Source: CAD feature listing. Evaluate the final solid. Frame: model axes, mm. A direction names the side the tool comes from. Give positions to 0.01 mm unless a question says otherwise; leave off trailing zeros. Write each loop counter-clockwise with the first axis right and the second up, starting at its lowest first coordinate (ties: lowest second). Pieces come first, ordered by that corner, then holes. Notation, with made-up numbers: (75, 66) -> (120, 66) arc R25 ccw to (120, 99) -> close; hole circle Ø4 at (-23.75, 65). An arc over 180 degrees is marked (long way). Write item = value, one per line.
from build123d import *

# Parameters (mm, degrees)
SKETCH006_W     = 44
SKETCH006_H     = 43
SKETCH006_W_2   = 24
SKETCH006_H_2   = 23
PAD007_DEPTH    = 3
SKETCH007_W     = 44
SKETCH007_H     = 43
SKETCH007_W_2   = 38
SKETCH007_H_2   = 37
PAD008_DEPTH    = 40
CHAMFER007_SIZE = 1.9
CHAMFER008_SIZE = 0.4


with BuildPart() as part:
    # Sketch006 → Pad007 (new body)
    with BuildSketch(Plane.XY):
        Rectangle(SKETCH006_W, SKETCH006_H)
        Rectangle(SKETCH006_W_2, SKETCH006_H_2, mode=Mode.SUBTRACT)
    extrude(amount=PAD007_DEPTH)

    # Sketch007 (on Face9 of Pad007) → Pad008 (join)
    with BuildSketch(Plane(origin=(0, 0, 0), x_dir=(1, 0, 0), z_dir=(0, 0, -1))):
        Rectangle(SKETCH007_W, SKETCH007_H)
        Rectangle(SKETCH007_W_2, SKETCH007_H_2, mode=Mode.SUBTRACT)
    extrude(amount=PAD008_DEPTH)

    # Chamfer007
    chamfer007_edges = [part.edges().sort_by_distance(p)[0] for p in [
        (0, -11.5, 0),
        (12, 0, 0),
        (0, 11.5, 0),
        (-12, 0, 0),
    ]]
    chamfer(chamfer007_edges, length=CHAMFER007_SIZE)

    # Chamfer008
    chamfer008_edges = [part.edges().sort_by_distance(p)[0] for p in [
        (-22, 0, -40),
        (0, 21.5, -40),
        (22, 0, -40),
        (0, -21.5, -40),
        (-19, 0, -40),
        (0, 18.5, -40),
        (19, 0, -40),
        (0, -18.5, -40),
        (22, 21.5, -18.5),
        (-22, 21.5, -18.5),
        (0, 21.5, 3),
        (-22, 0, 3),
        (0, -21.5, 3),
        (22, 0, 3),
        (-12, 0, 3),
        (0, -11.5, 3),
        (12, 0, 3),
        (0, 11.5, 3),
        (-22, -21.5, -18.5),
        (22, -21.5, -18.5),
    ]]
    chamfer(chamfer008_edges, length=CHAMFER008_SIZE)


solid = part.part
1) Cut plane A-A (y = 4.5). Return the cut outline in (x, z).
Computed:
outline = (-22, -39.6) -> (-21.6, -40) -> (-19.4, -40) -> (-19, -39.6) -> (-19, 0) -> (-13.9, 0) -> (-12, 1.9) -> (-12, 2.6) -> (-12.4, 3) -> (-21.6, 3) -> (-22, 2.6) -> close; (12, 1.9) -> (13.9, 0) -> (19, 0) -> (19, -39.6) -> (19.4, -40) -> (21.6, -40) -> (22, -39.6) -> (22, 2.6) -> (21.6, 3) -> (12.4, 3) -> (12, 2.6) -> close
2) Cut plane C-C (z = -2). Return the cut outline in (x, y).
Computed:
outline = (-22, -21.1) -> (-21.6, -21.5) -> (21.6, -21.5) -> (22, -21.1) -> (22, 21.1) -> (21.6, 21.5) -> (-21.6, 21.5) -> (-22, 21.1) -> close; hole (-19, -18.5) -> (19, -18.5) -> (19, 18.5) -> (-19, 18.5) -> close
3) Draft query along Y for faces 1 (the flat face through (-2, 20, -40)), 2 (the flat face through (0, -21.5, -18)), 3 (the flat face through (19, 0, -20)), 4 (the flat face through (-0.2, -12.4, 1)). Return one class per face: pulls with the +Y half, pulls with the -Y half, needs draft (parallel to the pull), parting line crosses it, or undercut.
Computed:
face_1 = needs draft
face_2 = pulls with the -Y half
face_3 = undercut
face_4 = undercut
4) Contact query for a flat-ended pin moving along its axis: pin 1 (1.5 mm diameter, centred on x = 14.5, y = 9.5, fed in from -Z). Output: stop coordinate, or through.
Computed:
pin_1 = 0
5) Cut plane D-D (x = 18). Return the cut outline in (y, z).
Computed:
outline = (-21.5, -39.6) -> (-21.1, -40) -> (-18.9, -40) -> (-18.5, -39.6) -> (-18.5, 0) -> (18.5, 0) -> (18.5, -39.6) -> (18.9, -40) -> (21.1, -40) -> (21.5, -39.6) -> (21.5, 2.6) -> (21.1, 3) -> (-21.1, 3) -> (-21.5, 2.6) -> close
6) Material intervals for L1, parallel to X at y = -2, z = -32; L2, parallel to Y at x = 15, z = -7.5; L3, parallel to Z at x = -2, y = -16.5, sorted ascending.
Computed:
L1 = -22 to -19, 19 to 22
L2 = -21.5 to -18.5, 18.5 to 21.5
L3 = 0 to 3
7) Cut plane B-B (x = -5). Return the cut outline in (y, z), then the cut area to 3 significant figures.
Computed:
outline = (-21.5, -39.6) -> (-21.1, -40) -> (-18.9, -40) -> (-18.5, -39.6) -> (-18.5, 0) -> (-13.4, 0) -> (-11.5, 1.9) -> (-11.5, 2.6) -> (-11.9, 3) -> (-21.1, 3) -> (-21.5, 2.6) -> close; (11.5, 1.9) -> (13.4, 0) -> (18.5, 0) -> (18.5, -39.6) -> (18.9, -40) -> (21.1, -40) -> (21.5, -39.6) -> (21.5, 2.6) -> (21.1, 3) -> (11.9, 3) -> (11.5, 2.6) -> close
area = 296 mm²
8) Access query for faces 5 (the flat face through (0, 21.5, -18)), 6 (the flat face through (0, -16, 0)). Directions: +Z, -Z, +X, -X, +Y, -Y. A direction counts if a zero-diameter tool reaches every point of the face in a straight line with its end or side. Return the directions, or none.
Computed:
face_5 = +Z, -Z, +X, -X, +Y
face_6 = -Z
